Could you check a few things on this drawing? It's one solid part, dimensions in mm from its lowest x, y, z. A direction names the side the tool comes from. Give positions to 0.01 mm unless a question says otherwise; leave off trailing zeros. Loops run counter-clockwise (first coordinate to the right, second up) from the corner with the lowest first, then second, coordinate; pieces in that order, holes last. Notation, with made-up numbers: (47.25, -7) - (92.25, -7) arc R31 ccw to (92.25, 28) - close; hole circle Ø9 at (68, 75.25). An arc over 180 degrees is marked (long way). Return JSON: item names as keys, results as strings. Group by question number.
(1) If we section it at A-A (x = 3): Please give me the cut outline in (y, z), then the cut area to 3 significant figures.
(2) For P1, Ø3, axis at x = 4, y = 5, coming from the -Z side, with a flat end and sliding along its axis, tell me the tip position at first contact or that it passes through.
(3) If we mould it in two halves opening along Z, with no side actions, what happens to the marked faces 1, 2 and 3? For each: released by +Z, released by -Z, zero draft, split by the parting line, or undercut.
(4) If we section it at C-C (y = 9.75): Please give me the cut outline in (x, z).
(5) On a 3-axis mill with a long thin cutter (end or side, diameter ignored), from which of +Z, -Z, +X, -X, +Y, -Y can I reach the whole of each face in a straight line? I mean the marked faces 4 and 5. Say none if no direction works.
(6) If we section it at B-B (y = 18.5): Please give me the cut outline in (x, z).
(7) I need wall thicknesses on probe 1 along Z at (x, y) = (3, 8.75); probe 2 along X at (y, z) = (18.25, 3.35) (1 decimal); probe 3 along X at (y, z) = (3, 2.7). Which ranges of each line are inside material? Lowest first, please. Write a range as [from, to].
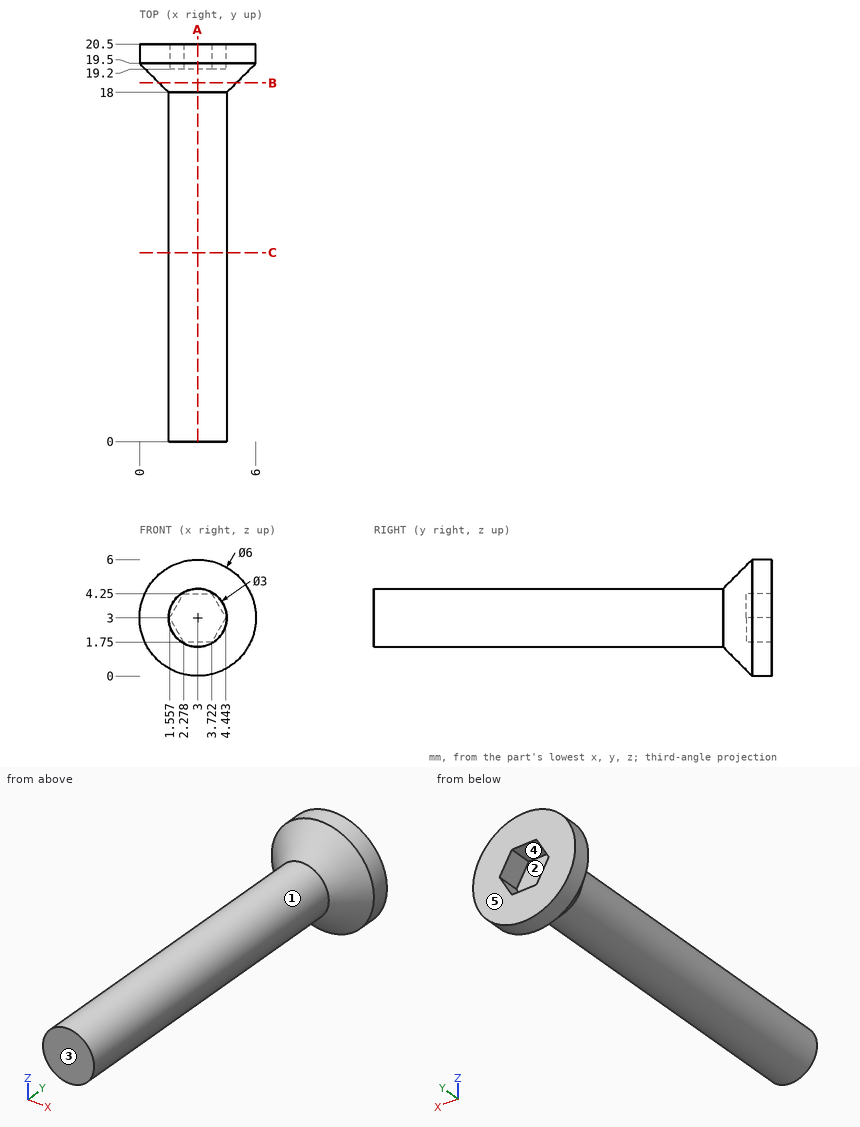
Values:
{
 "1": {"outline": "(0, 1.5) - (18, 1.5) - (19.5, 0) - (20.5, 0) - (20.5, 1.75) - (19.2, 1.75) - (19.2, 4.25) - (20.5, 4.25) - (20.5, 6) - (19.5, 6) - (18, 4.5) - (0, 4.5) - close", "area": "63.5 mm2"},
 "2": {"P1": "z = 1.5"},
 "3": {"face 1": "split by the parting line", "face 2": "undercut", "face 3": "zero draft"},
 "4": {"outline": "circle Ø3 at (3, 3)"},
 "5": {"face 4": "+Y", "face 5": "+Z, -Z, +X, -X, +Y"},
 "6": {"outline": "circle Ø4 at (3, 3)"},
 "7": {"probe 1": "[1.5, 4.5]", "probe 2": "[1.3, 4.7]", "probe 3": "[1.53, 4.47]"}
}
